Design review of the part built by this model. Coordinates are the model's own, in mm. A direction names the side the tool comes from. Coordinates: 2 decimals unless noted, no trailing zeros. Loops run counter-clockwise (first coordinate to the right, second up) from the corner with the lowest first, then second, coordinate; pieces in that order, holes last. Notation, with made-up numbers: (88.25, -38.75) - (95.25, -38.75) arc R23 cw to (95.25, -12.75) - close; hole circle Ø9 at (54, 80). An arc over 180 degrees is marked (long way). Answer in a Markdown table with one row per item. Add a question column.
(1) The part is to be moulded in two halves that separate along X. For faces 1 (the face through (0.1, -0.3, -45.7)), 2 (the face through (-5, 0, -38)), 3 (the face through (5, 0, 1)), say which applies: released by +X, released by -X, zero draft, split by the parting line, or undercut.
(2) For faces 4 (the face through (1.216, 1.115, 52.17)), 5 (the face through (2.5, -1.2, -9.6)), 6 (the face through (-4.43, -4.4, 0.81)), 7 (the face through (-2.535, -3.905, 15.133)), 8 (the face through (-1.216, 1.115, -52.17)), list the 3-axis set-ups (+Z, -Z, +X, -X, +Y, -Y) from which the entire face can be reached by the end or side of a thin tool; tool diameter is ignored.
(3) We need section B-B, the plane z = -31.5. Write out the cut boundary in (x, y), plus the area to 3 significant figures.
(4) Clearance check with flat-ended pins moving along their axes: pin 1 (6 mm diameter, centred on y = 0, z = 16, fed in from +X); pin 2 (2.5 mm diameter, centred on y = 0.5, z = 15, fed in from -X). State where each tip first meets the part, or that it passes through.
(5) We need section A-A, the plane z = 16. Write out the cut boundary in (x, y), plus the area to 3 significant figures.
(6) To check wall thickness, follow L1, parallel to Z at x = -2.8, y = 0; L2, parallel to Y at x = 1.95, z = -8; L3, parallel to X at y = 0, z = -51. State the ranges of each line that lie inside material, in increasing order. Write a range as [from, to].
from build123d import *

# Parameters (mm, degrees)
ESQUISSE1_W                                        = 10
ESQUISSE1_H                                        = 10
BOSS_EXTRU_1_DEPTH                                 = 58
CONG_1_R                                           = 2
TROU_TARAUD_M41_D                                  = 3.3
TROU_TARAUD_M41_DEPTH                              = 11.5
TROU_TARAUD_M41_TIP                                = 0.991420021
TROU_TARAUD_M42_D                                  = 3.3
TROU_TARAUD_M42_DEPTH                              = 11.5
TROU_TARAUD_M42_TIP                                = 0.991420021
DIAM_TRE_DU_PER_AGE_4_0_4_1_D                      = 4
DIAM_TRE_DU_PER_AGE_4_0_4_1_DEPTH                  = 5
DIAM_TRE_DU_PER_AGE_4_0_4_1_TIP                    = 1.201721238
CHAMBRAGE_POUR_VIS_T_TE_HEXAGONALE_M41_D           = 4.5
CHAMBRAGE_POUR_VIS_T_TE_HEXAGONALE_M41_CBORE_D     = 8
CHAMBRAGE_POUR_VIS_T_TE_HEXAGONALE_M41_CBORE_DEPTH = 5


with BuildPart() as part:
    # Esquisse1 → Boss.-Extru.1 (new, symmetric)
    with BuildSketch(Plane.XY):
        Rectangle(ESQUISSE1_W, ESQUISSE1_H)
    extrude(amount=BOSS_EXTRU_1_DEPTH, both=True)

    # Congé1
    cong_1_edges = [part.edges().sort_by_distance(p)[0] for p in [
        (-5, 5, 0),
        (5, 5, 0),
        (5, -5, 0),
        (-5, -5, 0),
    ]]
    fillet(cong_1_edges, radius=CONG_1_R)

    # Trou taraudé M41
    with Locations(Plane.XY.offset(58)):
        with Locations((0, 0)):
            Hole(TROU_TARAUD_M41_D / 2, depth=TROU_TARAUD_M41_DEPTH)
            with Locations((0, 0, -(TROU_TARAUD_M41_DEPTH + TROU_TARAUD_M41_TIP / 2))):  # 118° drill point
                Cone(0, TROU_TARAUD_M41_D / 2, TROU_TARAUD_M41_TIP, mode=Mode.SUBTRACT)

    # Trou taraudé M42
    with Locations(Plane(origin=(0, 0, -58), x_dir=(-1, 0, 0), z_dir=(0, 0, -1))):
        with Locations((0, 0)):
            Hole(TROU_TARAUD_M42_D / 2, depth=TROU_TARAUD_M42_DEPTH)
            with Locations((0, 0, -(TROU_TARAUD_M42_DEPTH + TROU_TARAUD_M42_TIP / 2))):  # 118° drill point
                Cone(0, TROU_TARAUD_M42_D / 2, TROU_TARAUD_M42_TIP, mode=Mode.SUBTRACT)

    # Diamètre du perçage Ø4.0 (4)1
    with Locations(Plane(origin=(5, 0, 0), x_dir=(0, 0, -1), z_dir=(1, 0, 0))):
        with Locations((8, 0), (-8, 0)):
            Hole(DIAM_TRE_DU_PER_AGE_4_0_4_1_D / 2, depth=DIAM_TRE_DU_PER_AGE_4_0_4_1_DEPTH)
            with Locations((0, 0, -(DIAM_TRE_DU_PER_AGE_4_0_4_1_DEPTH + DIAM_TRE_DU_PER_AGE_4_0_4_1_TIP / 2))):  # 118° drill point
                Cone(0, DIAM_TRE_DU_PER_AGE_4_0_4_1_D / 2, DIAM_TRE_DU_PER_AGE_4_0_4_1_TIP, mode=Mode.SUBTRACT)

    # Chambrage pour vis à tête hexagonale M41 (through all)
    with Locations(Plane.ZY.offset(5)):
        with Locations((-16, 0), (16, 0)):
            CounterBoreHole(CHAMBRAGE_POUR_VIS_T_TE_HEXAGONALE_M41_D / 2, CHAMBRAGE_POUR_VIS_T_TE_HEXAGONALE_M41_CBORE_D / 2, CHAMBRAGE_POUR_VIS_T_TE_HEXAGONALE_M41_CBORE_DEPTH)


solid = part.part
Responses:
| question | item | result |
|---|---|---|
| 1 | face 1 | undercut |
| 1 | face 2 | released by -X |
| 1 | face 3 | released by +X |
| 2 | face 4 | +Z |
| 2 | face 5 | +X |
| 2 | face 6 | +Z, -Z, -X, -Y |
| 2 | face 7 | -X |
| 2 | face 8 | -Z |
| 3 | outline | (-5, -3) arc R2 ccw to (-3, -5) - (3, -5) arc R2 ccw to (5, -3) - (5, 3) arc R2 ccw to (3, 5) - (-3, 5) arc R2 ccw to (-5, 3) - close |
| 3 | area | 96.6 mm2 |
| 4 | pin 1 | stops at x = 5 |
| 4 | pin 2 | stops at x = 0 |
| 5 | outline | (-4.73, -4) arc R2 ccw to (-3, -5) - (3, -5) arc R2 ccw to (5, -3) - (5, -2.25) - (0, -2.25) - (0, -4) - close; (-4.73, 4) - (0, 4) - (0, 2.25) - (5, 2.25) - (5, 3) arc R2 ccw to (3, 5) - (-3, 5) arc R2 ccw to start |
| 5 | area | 34.2 mm2 |
| 6 | L1 | z = [-58, -20], [-12, 12], [20, 58] |
| 6 | L2 | y = [-5, -2], [2, 5] |
| 6 | L3 | x = [-5, -1.65], [1.65, 5] |
